from build123d import *

# Parameters (mm, degrees)
SKETCH_1_R          = 4
EXTRUDE_1_DEPTH     = 11
SKETCH_2_R          = 3
EXTRUDE_2_DEPTH     = 8
CUT_EXTRUDE_START   = 5.2
SKETCH_3_OUTSIDE_W  = 16.412
SKETCH_3_OUTSIDE_H  = 16.412
SKETCH_3_OUTSIDE_R  = 2.75
CUT_EXTRUDE_1_DEPTH = 1.5
CHAMFER_1_SIZE      = 0.5


with BuildPart() as part:
    # 草图1 → 凸台-拉伸1 (new, symmetric)
    with BuildSketch(Plane(origin=(0, 0, 0), x_dir=(1, 0, 0), z_dir=(0, 1, 0))):
        with Locations(Location((0, 0, 0), (0, 0, 270))):
            Circle(SKETCH_1_R)
    extrude(amount=EXTRUDE_1_DEPTH, both=True)

    # 草图2 → 凸台-拉伸2 (add)
    with BuildSketch(Plane(origin=(0, 11, 0), x_dir=(1, 0, 0), z_dir=(0, 1, 0))):
        with Locations(Location((0, 0, 0), (0, 0, 270))):
            Circle(SKETCH_2_R)
    extrude(amount=EXTRUDE_2_DEPTH)

    # 草图3 outside → 切除-拉伸1 (cut)
    with BuildSketch(Plane(origin=(0, 11, 0), x_dir=(1, 0, 0), z_dir=(0, 1, 0)).offset(CUT_EXTRUDE_START)):
        Rectangle(SKETCH_3_OUTSIDE_W, SKETCH_3_OUTSIDE_H)
        with Locations(Location((0, 0, 0), (0, 0, 270))):
            Circle(SKETCH_3_OUTSIDE_R, mode=Mode.SUBTRACT)
    extrude(amount=CUT_EXTRUDE_1_DEPTH, mode=Mode.SUBTRACT)

    # 倒角1
    chamfer_1_edges = [part.edges().sort_by_distance(p)[0] for p in [
        (0, 19, -3),
    ]]
    chamfer(chamfer_1_edges, length=CHAMFER_1_SIZE)


solid = part.part
Input: part model. Units: mm. Frame: model coordinates. A direction names the side the tool comes from. Coordinates: 2 decimals unless noted, no trailing zeros. Order: outer loops, then holes, each group sorted by start corner. A loop starts at its lowest first (then second) coordinate and runs counter-clockwise, first axis right, second up. Notation, with made-up numbers: M 44,56.25 L 81,56.25 A33 ccw 81,85.25 Z; hole C -14,26 d11. An arc over 180 degrees is marked long. Write item = value, one per line. Start each with the question number.
(1) Reachability of faces 1 (the flat face through (0, -11, 0)), 2 (the cylindrical face through (0.9, 13.56, 2.86)), 3 (the cylindrical face through (-2.685, 16.94, -0.596)) from +Z, -Z, +X, -X, +Y, -Y: full face, straight path, thin tool, end or side. Return the list, or none.
(2) Section B-B on y = -6.75. Output: boundary loops of the cut face in (x, z).
(3) Section A-A on z = 0. Output: boundary loops of the cut face in (x, y).
(4) First-contact query: P1, Ø1.5, axis at y = 9, z = 1, coming from the +X side; P2, Ø4, axis at y = 14.5, z = -2.5, coming from the -X side. Flat tips, straight axial feed; report the tip coordinate or a pass-through.
(5) Line query: line 1 along Y through (x, z) = (-0.25, 3.25); line 2 along Z through (x, y) = (0, 13); line 3 along Z through (x, y) = (3, 6.25). Output: solid intervals per line, ascending. Write a range as [from, to].
Result set:
q1.face_1 = +Z, -Z, +X, -X, -Y
q1.face_2 = +Y
q1.face_3 = none
q2.outline = C 0,0 d8
q3.outline = M -4,-11 L 4,-11 L 4,11 L 3,11 L 3,16.2 L 2.75,16.2 L 2.75,17.7 L 3,17.7 L 3,18.5 L 2.5,19 L -2.5,19 L -3,18.5 L -3,17.7 L -2.75,17.7 L -2.75,16.2 L -3,16.2 L -3,11 L -4,11 Z
q4.P1 = 3.99
q4.P2 = -2.96
q5.line_1 = [-11, 11]
q5.line_2 = [-3, 3]
q5.line_3 = [-2.65, 2.65]
